```python
from build123d import *

# Parameters (mm, degrees)
SKETCH3_R          = 2.5796875
RIGHT_LEAF_DEPTH   = 50.0065
SKETCH11_R         = 3
CUT_EXTRUDE1_DEPTH = 10
CUT_EXTRUDE2_DEPTH = 24
CUT_EXTRUDE5_DEPTH = 24


with BuildPart() as part:
    # Sketch3 → Right Leaf (new, symmetric)
    with BuildSketch(Plane(origin=(0, 0, 0), x_dir=(0, 0, -1), z_dir=(1, 0, 0))):
        with BuildLine():
            Line((5.474302966, -8), (30.1625, -8))
            Line((30.1625, -8), (30.1625, -4.5202))
            Line((30.1625, -4.5202), (7.045897034, -4.5202))
            Line((7.045897034, -4.5202), (5.425308633, -2.899611599))
            ThreePointArc((5.425308633, -2.899611599), (-4.349811559, 4.349811559), (2.899611599, -5.425308633))
            Line((2.899611599, -5.425308633), (5.474302966, -8))
        make_face()
        Circle(SKETCH3_R, mode=Mode.SUBTRACT)
    extrude(amount=RIGHT_LEAF_DEPTH, both=True)

    # Sketch11 → Cut-Extrude1 (cut)
    with BuildSketch(Plane(origin=(0, -4.5202, 0), x_dir=(1, 0, 0), z_dir=(0, 1, 0))):
        with Locations(Location((-35.0065, 20.1625, 0), (0, 0, 270))):
            Circle(SKETCH11_R)
        with Locations(Location((-0.0065, 20.1625, 0), (0, 0, 270))):
            Circle(SKETCH11_R)
        with Locations(Location((34.9935, 20.1625, 0), (0, 0, 270))):
            Circle(SKETCH11_R)
    extrude(amount=-CUT_EXTRUDE1_DEPTH, mode=Mode.SUBTRACT)

    # Sketch12 → Cut-Extrude2 (cut)
    with BuildSketch(Plane(origin=(36.0065, 0, 0), x_dir=(0, 0, -1), z_dir=(1, 0, 0))):
        with BuildLine():
            Line((2.899611599, -5.425308633), (5.474302966, -8))
            Line((5.474302966, -8), (7.045897034, -8))
            Line((7.045897034, -8), (7.045897034, -4.5202))
            Line((7.045897034, -4.5202), (5.425308633, -2.899611599))
            ThreePointArc((5.425308633, -2.899611599), (-4.349811559, 4.349811559), (2.899611599, -5.425308633))
        make_face()
    extrude(amount=-CUT_EXTRUDE2_DEPTH, mode=Mode.SUBTRACT)

    # Sketch14 → Cut-Extrude5 (cut)
    with BuildSketch(Plane.ZY.offset(11.9935)):
        with BuildLine():
            Line((-5.425308633, -2.899611599), (-7.045897034, -4.5202))
            Line((-7.045897034, -4.5202), (-7.045897034, -8))
            Line((-7.045897034, -8), (-5.474302966, -8))
            Line((-5.474302966, -8), (-2.899611599, -5.425308633))
            ThreePointArc((-2.899611599, -5.425308633), (4.349811559, 4.349811559), (-5.425308633, -2.899611599))
        make_face()
    extrude(amount=CUT_EXTRUDE5_DEPTH, mode=Mode.SUBTRACT)


solid = part.part
```
For this review, take the finished solid that the model builds, in its own axes (mm). A direction names the side the tool comes from. Give positions to 0.01 mm unless a question says otherwise; leave off trailing zeros. Loops run counter-clockwise (first coordinate to the right, second up) from the corner with the lowest first, then second, coordinate; pieces in that order, holes last. Notation, with made-up numbers: M 78.25,-13.75 L 96.25,-13.75 A20 ccw 96.25,9.25 Z; hole C 6.5,77 d11. An arc over 180 degrees is marked long. One line per item, written item: value. Start each with the question number.
Q1. For L1, parallel to X at y = -6, z = -20; L2, parallel to Y at x = -39.75, z = 0; L3, parallel to X at y = 5.25, z = -3, list the stretches that pass through material, from the lowest coordinate up.
Q2. Machinability: for faces 1 (the face through (-11.994, -2, -2)), 2 (the face through (0.175, -6.695, -4.169)), 3 (the face through (43.104, -3.721, -6.247)), which of the approach directions +Z, -Z, +X, -X, +Y, -Y give a long, thin tool a straight path to every point of the face, cutting with its end or side? Answer none if there is none.
Q3. Add section C-C (x = 4). Give the boundary of the cut face in (y, z).
Q4. Draft analysis for pull direction Y (two halves, no side actions). For faces 4 (the face through (-0.16, -2.52, 0.56)), 5 (the face through (-43.1, -2.52, 0.56)), 6 (the face through (-24, -6, -7.046)), 7 (the face through (1, -4.52, -16)), state which applies: released by +Y, released by -Y, zero draft, split by the parting line, or undercut.
Q5. Add section A-A (y = 0). Give the boundary of the cut face in (x, z).
Q6. Clearance check with flat-ended pins moving along their axes: pin 1 Ø6 at (x, z) = (14.5, -19) entering from +Y; pin 2 Ø1.7 at (x, y) = (24, -6.5) entering from +Z; pin 3 Ø8 at (x, y) = (6.5, -6.5) entering from +Z. State where each tip first meets the part, or that it passes through.
Q7. Add section D-D (y = 5). Give the boundary of the cut face in (x, z).
Reply:
1. L1: -50.01 to -38, -32.01 to -3, 2.99 to 32, 37.99 to 50.01
1. L2: -6.15 to -2.58, 2.58 to 6.15
1. L3: -50.01 to -35.99, -11.99 to 12.01, 36.01 to 50.01
2. face 1: +Z, +Y, -Y
2. face 2: +X, -X, -Y
2. face 3: -Z, +X, -X
3. outline: M -8,-30.16 L -4.52,-30.16 L -4.52,-7.05 L -2.9,-5.43 A6.15 ccw long -5.43,-2.9 L -8,-5.47 Z; hole C 0,0 d5.16
4. face 4: undercut
4. face 5: undercut
4. face 6: zero draft
4. face 7: released by +Y
5. outline: M -50.01,-6.15 L -35.99,-6.15 L -35.99,-2.58 L -50.01,-2.58 Z; M -50.01,2.58 L -35.99,2.58 L -35.99,6.15 L -50.01,6.15 Z; M -11.99,-6.15 L 12.01,-6.15 L 12.01,-2.58 L -11.99,-2.58 Z; M -11.99,2.58 L 12.01,2.58 L 12.01,6.15 L -11.99,6.15 Z; M 36.01,-6.15 L 50.01,-6.15 L 50.01,-2.58 L 36.01,-2.58 Z; M 36.01,2.58 L 50.01,2.58 L 50.01,6.15 L 36.01,6.15 Z
6. pin 1: y = -4.52
6. pin 2: z = -7.05
6. pin 3: z = 5.62
7. outline: M -50.01,-3.58 L -35.99,-3.58 L -35.99,3.58 L -50.01,3.58 Z; M -11.99,-3.58 L 12.01,-3.58 L 12.01,3.58 L -11.99,3.58 Z; M 36.01,-3.58 L 50.01,-3.58 L 50.01,3.58 L 36.01,3.58 Z
